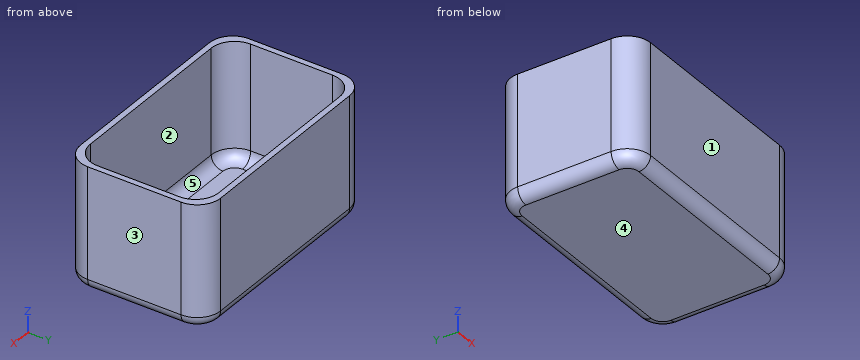
```python
from build123d import *

# Parameters (mm, degrees)
F1_DEPTH = 3.175
F2_DEPTH = 63.5
F3_R     = 6.35


with BuildPart() as f1:
    # F0 (on Top) → F1 (new body)
    with BuildSketch(Plane.XY):
        with BuildLine():
            ThreePointArc((63.5, 25.4), (59.7802561211, 34.3802561211), (50.8, 38.1))
            Line((50.8, 38.1), (-50.8, 38.1))
            ThreePointArc((-50.8, 38.1), (-59.7802561211, 34.3802561211), (-63.5, 25.4))
            Line((-63.5, 25.4), (-63.5, -25.4))
            ThreePointArc((-63.5, -25.4), (-59.7802561211, -34.3802561211), (-50.8, -38.1))
            Line((-50.8, -38.1), (50.8, -38.1))
            ThreePointArc((50.8, -38.1), (59.7802561211, -34.3802561211), (63.5, -25.4))
            Line((63.5, -25.4), (63.5, 25.4))
        make_face()
        with BuildLine():
            Line((-47.625, 34.925), (47.625, 34.925))
            ThreePointArc((47.625, 34.925), (56.6052561211, 31.2052561211), (60.325, 22.225))
            Line((60.325, 22.225), (60.325, -22.225))
            ThreePointArc((60.325, -22.225), (56.6052561211, -31.2052561211), (47.625, -34.925))
            Line((47.625, -34.925), (-47.625, -34.925))
            ThreePointArc((-47.625, -34.925), (-56.6052561211, -31.2052561211), (-60.325, -22.225))
            Line((-60.325, -22.225), (-60.325, 22.225))
            ThreePointArc((-60.325, 22.225), (-56.6052561211, 31.2052561211), (-47.625, 34.925))
        make_face(mode=Mode.SUBTRACT)
        with BuildLine():
            ThreePointArc((60.325, 22.225), (56.6052561211, 31.2052561211), (47.625, 34.925))
            Line((47.625, 34.925), (-47.625, 34.925))
            ThreePointArc((-47.625, 34.925), (-56.6052561211, 31.2052561211), (-60.325, 22.225))
            Line((-60.325, 22.225), (-60.325, -22.225))
            ThreePointArc((-60.325, -22.225), (-56.6052561211, -31.2052561211), (-47.625, -34.925))
            Line((-47.625, -34.925), (47.625, -34.925))
            ThreePointArc((47.625, -34.925), (56.6052561211, -31.2052561211), (60.325, -22.225))
            Line((60.325, -22.225), (60.325, 22.225))
        make_face()
    extrude(amount=-F1_DEPTH)

    # F0 (on Top) → F2 (join)
    with BuildSketch(Plane.XY):
        with BuildLine():
            ThreePointArc((63.5, 25.4), (59.7802561211, 34.3802561211), (50.8, 38.1))
            Line((50.8, 38.1), (-50.8, 38.1))
            ThreePointArc((-50.8, 38.1), (-59.7802561211, 34.3802561211), (-63.5, 25.4))
            Line((-63.5, 25.4), (-63.5, -25.4))
            ThreePointArc((-63.5, -25.4), (-59.7802561211, -34.3802561211), (-50.8, -38.1))
            Line((-50.8, -38.1), (50.8, -38.1))
            ThreePointArc((50.8, -38.1), (59.7802561211, -34.3802561211), (63.5, -25.4))
            Line((63.5, -25.4), (63.5, 25.4))
        make_face()
        with BuildLine():
            Line((-47.625, 34.925), (47.625, 34.925))
            ThreePointArc((47.625, 34.925), (56.6052561211, 31.2052561211), (60.325, 22.225))
            Line((60.325, 22.225), (60.325, -22.225))
            ThreePointArc((60.325, -22.225), (56.6052561211, -31.2052561211), (47.625, -34.925))
            Line((47.625, -34.925), (-47.625, -34.925))
            ThreePointArc((-47.625, -34.925), (-56.6052561211, -31.2052561211), (-60.325, -22.225))
            Line((-60.325, -22.225), (-60.325, 22.225))
            ThreePointArc((-60.325, 22.225), (-56.6052561211, 31.2052561211), (-47.625, 34.925))
        make_face(mode=Mode.SUBTRACT)
    extrude(amount=F2_DEPTH)

    # F3
    f3_edges = [f1.edges().sort_by_distance(p)[0] for p in [
        (0, 34.925, 0),
        (0, -38.1, -3.175),
    ]]
    fillet(f3_edges, radius=F3_R)


solid = f1.part
```
Can you work these out from the model? Positions are in its coordinate system, mm. Face numbers are marked on the shaded views. A direction names the side the tool comes from. Coordinates: 2 decimals unless noted, no trailing zeros. Loops run counter-clockwise (first coordinate to the right, second up) from the corner with the lowest first, then second, coordinate; pieces in that order, holes last. Notation, with made-up numbers: (10, 6) - (24, 6) arc R16 ccw to (24, 19) - close; hole circle Ø4 at (15.25, 14.25). An arc over 180 degrees is marked (long way). Answer as CSV lines item,"result". Start each with the question number.
1) Suppose I cut it at A-A (z = 58). Please give me the cut outline in (x, y) (3 decimals).
2) Thinking about a two-plate mould opening in X: for the marked faces 1, 2 and 3, which applies, pulls with the +X half, pulls with the -X half, needs draft (parallel to the pull), parting line crosses it, or undercut?
3) Suppose I cut it at B-B (x = -13). Please give me the cut outline in (y, z) (3 decimals), plus the area to 3 significant figures.
4) Suppose I cut it at C-C (y = -10). Please give me the cut outline in (x, z) (3 decimals), plus the area to 3 significant figures.
5) For pin 1 (5 mm diameter, centred on x = -31, y = 5.5, fed in from +Z), with a flat end and sliding along its axis, tell me the tip position at first contact or that it passes through.
6) Which directions (+Z, -Z, +X, -X, +Y, -Y) give clear straight access to the entire face, cutting with the end or side of a thin tool? Please do the marked faces 4 and 5.
7) I need wall thicknesses on line 1 (Y direction, x = 43.5, z = 21) (3 decimals); line 2 (X direction, y = 20, z = 55.5) (3 decimals); line 3 (Z direction, x = -49, y = 6) (3 decimals). Which ranges of each line are inside material? Lowest first, please. Write a range as from..to.
Check result:
1,outline,"(-63.5, -25.4) arc R12.7 ccw to (-50.8, -38.1) - (50.8, -38.1) arc R12.7 ccw to (63.5, -25.4) - (63.5, 25.4) arc R12.7 ccw to (50.8, 38.1) - (-50.8, 38.1) arc R12.7 ccw to (-63.5, 25.4) - close; hole (-60.325, -22.225) arc R12.7 ccw to (-47.625, -34.925) - (47.625, -34.925) arc R12.7 ccw to (60.325, -22.225) - (60.325, 22.225) arc R12.7 ccw to (47.625, 34.925) - (-47.625, 34.925) arc R12.7 ccw to (-60.325, 22.225) - close"
2,face 1,"needs draft"
2,face 2,"undercut"
2,face 3,"pulls with the +X half"
3,outline,"(-38.1, 3.175) arc R6.35 ccw to (-31.75, -3.175) - (31.75, -3.175) arc R6.35 ccw to (38.1, 3.175) - (38.1, 63.5) - (34.925, 63.5) - (34.925, 6.35) arc R6.35 cw to (28.575, 0) - (-28.575, 0) arc R6.35 cw to (-34.925, 6.35) - (-34.925, 63.5) - (-38.1, 63.5) - close"
3,area,"645 mm²"
4,outline,"(-63.5, 3.175) arc R6.35 ccw to (-57.15, -3.175) - (57.15, -3.175) arc R6.35 ccw to (63.5, 3.175) - (63.5, 63.5) - (60.325, 63.5) - (60.325, 6.35) arc R6.35 cw to (53.975, 0) - (-53.975, 0) arc R6.35 cw to (-60.325, 6.35) - (-60.325, 63.5) - (-63.5, 63.5) - close"
4,area,"806 mm²"
5,pin 1,"stops at z = 0"
6,face 4,"-Z, +X, -X, +Y, -Y"
6,face 5,"+Z"
7,line 1,"y = -38.1..-34.925, 34.925..38.1"
7,line 2,"x = -63.5..-60.325, 60.325..63.5"
7,line 3,"z = -3.175..0"
